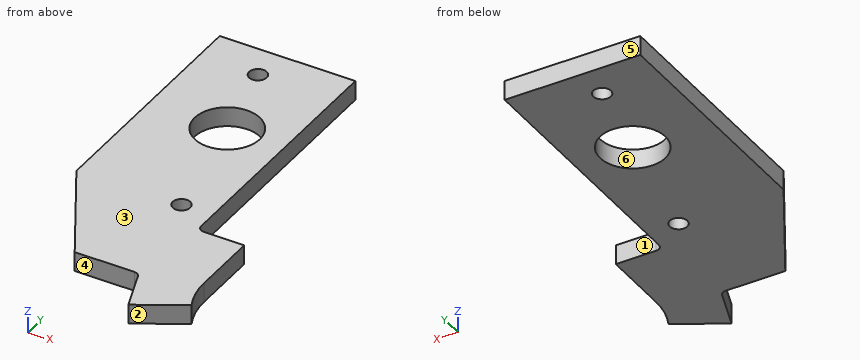
from build123d import *

# Parameters (mm, degrees)
BOSS_EXTRUDE1_DEPTH          = 4.7625
F_6_CLEARANCE_HOLE1_D        = 4.3053
F_5_8_0_625_DIAMETER_HOLE1_D = 15.875


with BuildPart() as part:
    # Sketch1 → Boss-Extrude1 (new body)
    with BuildSketch(Plane.XY):
        with BuildLine():
            Line((-3163.88635614, 1099.09115169), (-3160.187774322, 1088.929381663))
            Line((-3160.187774322, 1088.929381663), (-3148.734838552, 1095.541737213))
            ThreePointArc((-3148.734838552, 1095.541737213), (-3150.193848799, 1099.631639206), (-3150.688757178, 1103.945694712))
            Line((-3150.688757178, 1103.945694712), (-3150.688757178, 1120.455694712))
            Line((-3150.688757178, 1120.455694712), (-3160.531257178, 1120.455694712))
            ThreePointArc((-3160.531257178, 1120.455694712), (-3161.653789193, 1120.920662697), (-3162.118757178, 1122.043194712))
            Line((-3162.118757178, 1122.043194712), (-3162.118757178, 1185.225694712))
            Line((-3162.118757178, 1185.225694712), (-3195.138757178, 1185.225694712))
            Line((-3195.138757178, 1185.225694712), (-3195.138757178, 1126.488194712))
            Line((-3195.138757178, 1126.488194712), (-3179.898757178, 1100.135694712))
            Line((-3179.898757178, 1100.135694712), (-3165.378118175, 1100.135694712))
            ThreePointArc((-3165.378118175, 1100.135694712), (-3164.467565582, 1099.848598583), (-3163.88635614, 1099.09115169))
        make_face()
    extrude(amount=BOSS_EXTRUDE1_DEPTH)

    # #6 Clearance Hole1 (through all)
    with Locations(Plane.XY.offset(4.7625)):
        with Locations((-3169.738757178, 1126.805694712), (-3180.851257178, 1176.843694712)):
            Hole(F_6_CLEARANCE_HOLE1_D / 2)

    # 5/8 (0.625) Diameter Hole1 (through all)
    with Locations(Plane.XY.offset(4.7625)):
        with Locations((-3176.088757178, 1156.269694712)):
            Hole(F_5_8_0_625_DIAMETER_HOLE1_D / 2)


solid = part.part
Work out the finished part from the listing and answer in its coordinate system (mm). Face numbers are marked on the shaded views. A direction names the side the tool comes from. Round coordinates to 2 decimals unless told otherwise and drop trailing zeros. Write each loop counter-clockwise with the first axis right and the second up, starting at its lowest first coordinate (ties: lowest second). Pieces come first, ordered by that corner, then holes.
1) A cutting plane is placed at C-C (y = 1133). Give the vertices of the cut face in (x, z).
2) A cutting plane is placed at A-A (x = -3176.5). Give the vertices of the cut face in (y, z).
3) A tool of negligible diameter and unlimited length cuts with its end or side. For the marked faces 1 and 2, from which of +Z, -Z, +X, -X, +Y, -Y can it reach the whole face along a straight path? Write none if from no direction.
4) A cutting plane is placed at D-D (x = -3156). Give the vertices of the cut face in (y, z).
5) The mould has two halves that part along Y. Classify the marked faces 3, 4, 5 and 6: pulls with the +Y half, pulls with the -Y half, needs draft (parallel to the pull), parting line crosses it, or undercut.
6) A cutting plane is placed at B-B (z = 3.55). Give the number of separate pieces and of enclosed holes in the cut face, plus the area to 3 significant figures.
7) Given pin 1 Ø2 at (y, z) = (1112.5, 1.5) entering from +X; pin 2 Ø1.4 at (y, z) = (1169, 2) entering from +X; pin 3 Ø14.5 at (x, y) = (-3176.09, 1156.27) entering from +Z; pin 4 Ø1.4 at (x, z) = (-3175.5, 2.5) entering from -Y, each flat-ended and moving along its own axis, determine where each tip first touches the part or whether it passes through.
8) Straight lines are drawn through the part: line 1 (Y direction, x = -3181.5, z = 1.55); line 2 (X direction, y = 1127, z = 3.9); line 3 (X direction, y = 1172.5, z = 1). For each, find the intervals that lie inside material, in ascending order.
Completed:
1. outline: (-3195.14, 0) - (-3162.12, 0) - (-3162.12, 4.76) - (-3195.14, 4.76) - close
2. outline: (1100.14, 0) - (1148.34, 0) - (1148.34, 4.76) - (1100.14, 4.76) - close; (1164.2, 0) - (1185.23, 0) - (1185.23, 4.76) - (1164.2, 4.76) - close
3. face 1: +Z, -Z, +X, +Y
3. face 2: +Z, -Z, +X, -Y
4. outline: (1091.35, 0) - (1120.46, 0) - (1120.46, 4.76) - (1091.35, 4.76) - close
5. face 3: needs draft
5. face 4: pulls with the -Y half
5. face 5: pulls with the +Y half
5. face 6: undercut
6. separate pieces: 1
6. enclosed holes: 3
6. area: 2,720 mm2
7. pin 1: stops at x = -3150.69
7. pin 2: stops at x = -3162.12
7. pin 3: passes through
7. pin 4: stops at y = 1100.14
8. line 1: y = 1102.9 to 1150.46, 1162.08 to 1174.79, 1178.9 to 1185.23
8. line 2: x = -3195.14 to -3171.88, -3167.59 to -3162.12
8. line 3: x = -3195.14 to -3162.12
